Verification items for this drawing (mm, ordinates from the low corner). A direction names the side the tool comes from. Coordinates: 2 decimals unless noted, no trailing zeros. Loops run counter-clockwise (first coordinate to the right, second up) from the corner with the lowest first, then second, coordinate; pieces in that order, holes last. Notation, with made-up numbers: (-8, 36.5) -> (36, 36.5) arc R20 ccw to (36, 65.5) -> close; hole circle Ø3 at (-12, -25). An arc over 180 degrees is marked (long way). Write item = value, one per line.
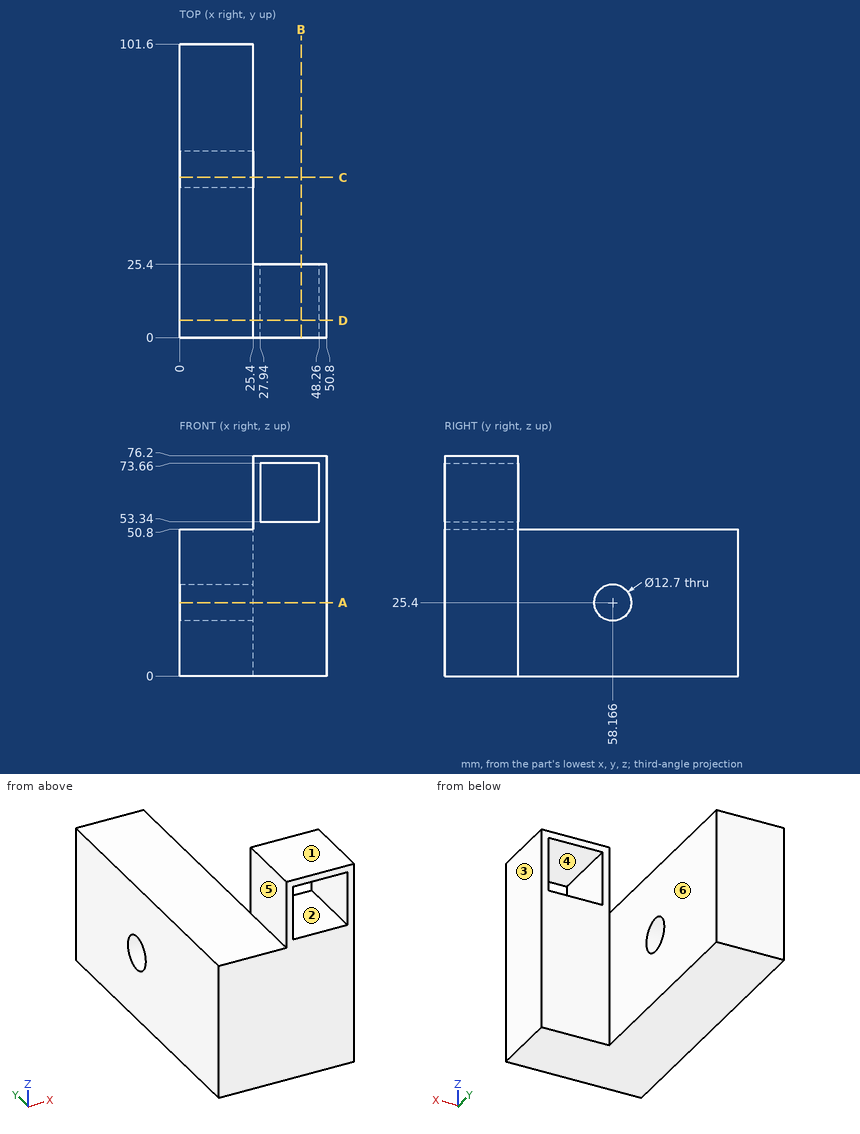
1) Release check for a two-part mould opening along X. For the marked faces 1, 2 and 3 record: pulls with the +X half, pulls with the -X half, needs draft (parallel to the pull), parting line crosses it, or undercut.
Ans:
face_1 = needs draft
face_2 = undercut
face_3 = pulls with the +X half
2) Material ranges on line 1 (X direction, y = 8, z = 59.5); line 2 (Y direction, x = 17.25, z = 25.4); line 3 (X direction, y = 33, z = 21), recorded low to high.
Ans:
line_1 = 25.4 to 27.94, 48.26 to 50.8
line_2 = 0 to 51.82, 64.52 to 101.6
line_3 = 0 to 25.4
3) Sectioned sample at A-A, the plane z = 25.4. Record the cut outline in (x, y).
Ans:
outline = (0, 0) -> (50.8, 0) -> (50.8, 25.4) -> (25.4, 25.4) -> (25.4, 51.82) -> (0, 51.82) -> close; (0, 64.52) -> (25.4, 64.52) -> (25.4, 101.6) -> (0, 101.6) -> close
4) Sectioned sample at D-D, the plane y = 6. Record the cut outline in (x, z), plus the area to 3 significant figures.
Ans:
outline = (0, 0) -> (50.8, 0) -> (50.8, 76.2) -> (25.4, 76.2) -> (25.4, 50.8) -> (0, 50.8) -> close; hole (27.94, 53.34) -> (48.26, 53.34) -> (48.26, 73.66) -> (27.94, 73.66) -> close
area = 2,810 mm2
5) Sectioned sample at B-B, the plane x = 42. Record the cut outline in (y, z), plus the area to 3 significant figures.
Ans:
outline = (0, 0) -> (25.4, 0) -> (25.4, 53.34) -> (0, 53.34) -> close; (0, 73.66) -> (25.4, 73.66) -> (25.4, 76.2) -> (0, 76.2) -> close
area = 1,420 mm2
6) Sectioned sample at C-C, the plane y = 55.5. Record the cut outline in (x, z), plus the area to 3 significant figures.
Ans:
outline = (0, 0) -> (25.4, 0) -> (25.4, 19.64) -> (0, 19.64) -> close; (0, 31.16) -> (25.4, 31.16) -> (25.4, 50.8) -> (0, 50.8) -> close
area = 998 mm2
7) Depth check by flat-ended pin: pin 1 Ø10 at (y, z) = (68, 12) entering from +X; pin 2 Ø7.5 at (y, z) = (15.5, 65.5) entering from -X; pin 3 Ø7.5 at (x, z) = (39, 38.5) entering from +Y. Enter the tip coordinate at first touch or a pass-through.
Ans:
pin_1 = 25.4
pin_2 = 25.4
pin_3 = 25.4
8) Tool access check on the marked faces 4, 5 and 6. Record the directions out of +Z, -Z, +X, -X, +Y, -Y that give a thin tool (end or side, any length) a straight path to the whole face; none if there is none.
Ans:
face_4 = +Y, -Y
face_5 = +Z, -X, +Y, -Y
face_6 = +Z, -Z, +X, +Y
